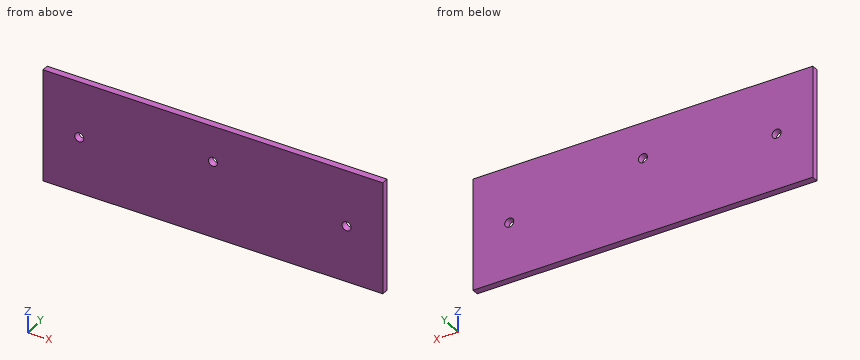
from build123d import *

# Parameters (mm, degrees)
SKETCH1_W           = 150
SKETCH1_H           = 50
BOSS_EXTRUDE1_DEPTH = 3
SKETCH2_R           = 2
CUT_EXTRUDE1_DEPTH  = 3
CUT_EXTRUDE2_REACH  = 5
SKETCH3_R           = 2


with BuildPart() as part:
    # Sketch1 → Boss-Extrude1 (new body)
    with BuildSketch(Plane(origin=(0, 0, 0), x_dir=(1, 0, 0), z_dir=(0, 1, 0))):
        Rectangle(SKETCH1_W, SKETCH1_H)
    extrude(amount=BOSS_EXTRUDE1_DEPTH)

    # Sketch2 → Cut-Extrude1 (cut)
    with BuildSketch(Plane(origin=(0, 3, 0), x_dir=(1, 0, 0), z_dir=(0, 1, 0))):
        with Locations(Location((59, 0, 0), (0, 0, 270))):  # turned: the seam where the file's is
            Circle(SKETCH2_R)
    cut_extrude1 = extrude(amount=-CUT_EXTRUDE1_DEPTH, mode=Mode.SUBTRACT)

    # Mirror1: Cut-Extrude1 across plane
    add(cut_extrude1.mirror(Plane(origin=(0, 0, 0), x_dir=(0, 0, 1), z_dir=(1, 0, 0))), mode=Mode.SUBTRACT)

    # Sketch3 → Cut-Extrude2 (cut, up to next)
    with BuildSketch(Plane(origin=(0, 3, 0), x_dir=(1, 0, 0), z_dir=(0, 1, 0)), mode=Mode.PRIVATE) as cut_extrude2_sk1:
        with Locations(Location((0, -9, 0), (0, 0, 270))):  # turned: the seam where the file's is
            Circle(SKETCH3_R)
    cut_extrude2_tool1 = extrude(cut_extrude2_sk1.sketch, amount=-CUT_EXTRUDE2_REACH, mode=Mode.PRIVATE) & part.part
    add(cut_extrude2_tool1.solids().sort_by_distance((0, 3, 9))[0], mode=Mode.SUBTRACT)


solid = part.part
Could you check a few things on this model? Use its own coordinates, in mm. Round coordinates to 2 decimals unless told otherwise and drop trailing zeros. Loops run counter-clockwise (first coordinate to the right, second up) from the corner with the lowest first, then second, coordinate; pieces in that order, holes last. Notation, with made-up numbers: (71, 38.5) - (96, 38.5) arc R4 cw to (96, 45.5) - close; hole circle Ø10 at (60, -14.75). An arc over 180 degrees is marked (long way). Write item = value, one per line.
1) I'm going to push a flat-ended pin straight in: P1, Ø2.5, axis at x = -59, z = 0, coming from the +Y side. Where does the tip first touch, or does it pass through?
Computed:
P1 = through
2) Imagine slicing it at B-B (x = -59). Please give me the cut outline in (y, z).
Computed:
outline = (0, -25) - (3, -25) - (3, -2) - (0, -2) - close; (0, 2) - (3, 2) - (3, 25) - (0, 25) - close
3) I need wall thicknesses on line 1 along X through (y, z) = (1.2, 0); line 2 along X through (y, z) = (1.3, 9); line 3 along X through (y, z) = (0.25, 1.5). Which ranges of each line are inside material? Lowest first, please. Write a range as from..to.
Computed:
line_1 = -75..-61, -57..57, 61..75
line_2 = -75..-2, 2..75
line_3 = -75..-60.32, -57.68..57.68, 60.32..75
4) Imagine slicing it at A-A (z = 0). Please give me the cut outline in (x, y), and give its area (3 significant figures).
Computed:
outline = (-75, 0) - (-61, 0) - (-61, 3) - (-75, 3) - close; (-57, 0) - (57, 0) - (57, 3) - (-57, 3) - close; (61, 0) - (75, 0) - (75, 3) - (61, 3) - close
area = 426 mm2
